from build123d import *

# Parameters (mm, degrees)
F1_DEPTH = 107.95
F2_R     = 5.715
F3_DEPTH = 5.08
F4_R     = 6.985
F5_DEPTH = 2.54
F7_DEPTH = 5.08


with BuildPart() as f1:
    # F0 (on Right) → F1 (new body)
    with BuildSketch(Plane.YZ):
        with BuildLine():
            Line((0, 10.16), (0, 1.27))
            ThreePointArc((0, 1.27), (0.371974, 0.371974), (1.27, 0))
            Line((1.27, 0), (1.905, 0))
            ThreePointArc((1.905, 0), (2.803026, 0.371974), (3.175, 1.27))
            Line((3.175, 1.27), (3.175, 9.525))
            ThreePointArc((3.175, 9.525), (3.972931, 11.858139), (6.0325, 13.214017))
            ThreePointArc((6.0325, 13.214017), (6.719023, 13.665976), (6.985, 14.443689))
            Line((6.985, 14.443689), (6.985, 15.24))
            ThreePointArc((6.985, 15.24), (6.613026, 16.138026), (5.715, 16.51))
            Line((5.715, 16.51), (1.27, 16.51))
            ThreePointArc((1.27, 16.51), (0.371974, 16.138026), (0, 15.24))
            Line((0, 15.24), (0, 10.16))
        make_face()
    extrude(amount=F1_DEPTH)

    # F2 (on face) → F3 (join)
    with BuildSketch(Plane.XZ):
        with BuildLine():
            ThreePointArc((53.975, 1.27), (58.914141, 3.315859), (60.96, 8.255))
            ThreePointArc((60.96, 8.255), (58.914141, 13.194141), (53.975, 15.24))
            ThreePointArc((53.975, 15.24), (46.99, 8.255), (53.975, 1.27))
        make_face()
        with Locations((53.975, 8.255)):
            Circle(F2_R, mode=Mode.SUBTRACT)
    extrude(amount=F3_DEPTH)

    # F4 (on face) → F5 (join)
    with BuildSketch(Plane.XZ.offset(5.08)):
        with Locations((53.975, 8.255)):
            Circle(F4_R)
    extrude(amount=F5_DEPTH)

    # F6 (on face) → F7 (cut)
    with BuildSketch(Plane.XZ.offset(7.62)):
        with BuildLine():
            Line((55.88, 13.335), (53.975, 13.335))
            Line((53.975, 13.335), (52.07, 13.335))
            ThreePointArc((52.07, 13.335), (50.273949, 12.591051), (49.53, 10.795))
            Line((49.53, 10.795), (49.53, 5.715))
            ThreePointArc((49.53, 5.715), (50.273949, 3.918949), (52.07, 3.175))
            Line((52.07, 3.175), (55.88, 3.175))
            ThreePointArc((55.88, 3.175), (57.676051, 3.918949), (58.42, 5.715))
            Line((58.42, 5.715), (58.42, 8.255))
            Line((58.42, 8.255), (58.42, 10.795))
            ThreePointArc((58.42, 10.795), (57.676051, 12.591051), (55.88, 13.335))
        make_face()
    extrude(amount=-F7_DEPTH, mode=Mode.SUBTRACT)


solid = f1.part
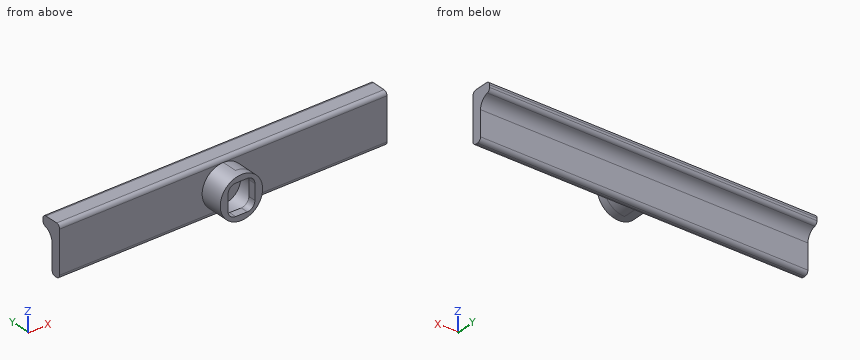
Check sheet for the modelled part. Datum: model origin and axes. Units: mm. Coordinates: 2 decimals unless noted, no trailing zeros. Write each loop counter-clockwise with the first axis right and the second up, starting at its lowest first coordinate (ties: lowest second). Pieces come first, ordered by that corner, then holes.
Item 1: Scan lines: probe 1 along Z at (x, y) = (31.5, 2); probe 2 along Y at (x, z) = (101, 8.5) (3 decimals); probe 3 along X at (y, z) = (-3, 10.5). Record each from-to range of solid material in increasing order.
Numbers:
probe 1: z = 0 to 16.51
probe 2: y = 0 to 3.175
probe 3: x = 47.36 to 48.72, 59.23 to 60.59
Item 2: Cross-section at B-B on x = 43.5. Record the boundary of the cut face in (y, z) (1 decimal).
Numbers:
outline: (0, 1.3) arc R1.3 ccw to (1.3, 0) - (1.9, 0) arc R1.3 ccw to (3.2, 1.3) - (3.2, 9.5) arc R3.8 cw to (6, 13.2) arc R1.3 ccw to (7, 14.4) - (7, 15.2) arc R1.3 ccw to (5.7, 16.5) - (1.3, 16.5) arc R1.3 ccw to (0, 15.2) - close
Item 3: Cross-section at A-A on y = -6.25. Record the boundary of the cut face in (x, z) (3 decimals).
Numbers:
outline: circle Ø13.97 at (53.975, 8.255); hole (49.53, 5.715) arc R2.54 ccw to (52.07, 3.175) - (55.88, 3.175) arc R2.54 ccw to (58.42, 5.715) - (58.42, 10.795) arc R2.54 ccw to (55.88, 13.335) - (52.07, 13.335) arc R2.54 ccw to (49.53, 10.795) - close
Item 4: Depth check by flat-ended pin: pin 1 Ø1.5 at (y, z) = (-4.5, 11) entering from -X; pin 2 Ø3 at (x, y) = (54, -6) entering from -Z; pin 3 Ø5 at (y, z) = (-4.5, 4) entering from +X. Enter the tip coordinate at first touch or a pass-through.
Numbers:
pin 1: stops at x = 47.28
pin 2: stops at z = 1.27
pin 3: stops at x = 60.74
